from build123d import *

# Parameters (mm, degrees)
F3_D            = 5.5
F3_COPIES_COUNT = 6


# Not quite as in the source:
# - a pattern or mirror of a feature is missing from the dataset's text; its kind, count and spacing are read off the source's solid


with BuildPart() as f1:
    # F0 (on Front) → F1 (revolve)
    with BuildSketch(Plane.XZ):
        Polygon((-25, 16.5), (-25, 11), (25, 11), (25, 16.5), (4, 18), (4, 34), (-4, 34), (-4, 18), align=None)
    revolve(axis=Axis((-2.8921069455, 0, 0), (1, 0, 0)))

    # F3 (through all)
    with Locations(Plane.YZ.offset(4)):
        with Locations((0, 25)):
            f3 = Hole(F3_D / 2)

    # F3_copies: F3 ×6 about axis
    f3_copies_axis = Axis((0, 0, 0), (1, 0, 0))
    for i in range(1, F3_COPIES_COUNT):
        add(f3.rotate(f3_copies_axis, i * 360 / F3_COPIES_COUNT), mode=Mode.SUBTRACT)


solid = f1.part
Design review of the part built by this model. Coordinates are the model's own, in mm. A direction names the side the tool comes from. Give positions to 0.01 mm unless a question says otherwise; leave off trailing zeros. Loops run counter-clockwise (first coordinate to the right, second up) from the corner with the lowest first, then second, coordinate; pieces in that order, holes last. Notation, with made-up numbers: (33.5, -12.5) - (53.5, -12.5) arc R33 cw to (53.5, 24.5) - close; hole circle Ø2 at (8, 43.25). An arc over 180 degrees is marked (long way). Use CSV: the item, a comma, the result in double quotes. Start each with the question number.
1. Insertion check: P1, Ø9, axis at y = 0, z = -25, coming from the +X side; P2, Ø9, axis at y = 0, z = 25, coming from the -X side; P3, Ø3, axis at x = 11.5, z = 7, coming from the -Y side. Each pin has a flat end and moves straight along its axis. Give the tip position at first contact, or say it passes through.
2. Machinability: for faces 4 (the cylindrical face through (-0.056, 0.358, 27.727)), 5 (the flat face through (4, 15, -15)), which of the approach directions +Z, -Z, +X, -X, +Y, -Y give a long, thin tool a straight path to every point of the face, cutting with its end or side? Answer none if there is none.
3. Add section A-A (z = 0). State the section outline as (x, y) points.
4. Draft analysis for pull direction Z (two halves, no side actions). For faces 1 (the conical face through (16.686, -5.135, 16.304)), 2 (the cylindrical face through (-0.056, -0.358, -27.727)), 3 (the flat face through (-4, 15, 15)), state which applies: released by +Z, released by -Z, zero draft, split by the parting line, or undercut.
5. Add section C-C (x = 20). State the section outline as (y, z) points, plus the area to 3 significant figures.
6. Add section D-D (z = 25). State the section outline as (x, y) points, plus the area to 3 significant figures.
7. Wall thickness on L1, parallel to Y at x = 1, z = 12; L2, parallel to X at y = -5, z = -19.5; L3, parallel to Y at x = 22.5, z = -1.5: over which ranges is each line inside the solid? List them lowest first.
8. Add section B-B (y = 0). State the section outline as (x, z) points.
Results found:
1,P1,"stops at x = 4"
1,P2,"stops at x = -4"
1,P3,"stops at y = -16.59"
2,face 4,"+X, -X"
2,face 5,"+X"
3,outline,"(-25, -16.5) - (-4, -18) - (-4, -34) - (4, -34) - (4, -18) - (25, -16.5) - (25, -11) - (-25, -11) - close; (-25, 11) - (25, 11) - (25, 16.5) - (4, 18) - (4, 34) - (-4, 34) - (-4, 18) - (-25, 16.5) - close"
4,face 1,"split by the parting line"
4,face 2,"undercut"
4,face 3,"zero draft"
5,outline,"circle Ø33.71 at (0, 0); hole circle Ø22 at (0, 0)"
5,area,"513 mm²"
6,outline,"(-4, -23.04) - (4, -23.04) - (4, -2.75) - (-4, -2.75) - close; (-4, 2.75) - (4, 2.75) - (4, 23.04) - (-4, 23.04) - close"
6,area,"325 mm²"
7,L1,"y = -31.81 to -24.35, -18.95 to 18.95, 24.35 to 31.81"
7,L2,"x = -4 to 4"
7,L3,"y = -16.61 to -10.9, 10.9 to 16.61"
8,outline,"(-25, -16.5) - (-4, -18) - (-4, -22.25) - (4, -22.25) - (4, -18) - (25, -16.5) - (25, -11) - (-25, -11) - close; (-25, 11) - (25, 11) - (25, 16.5) - (4, 18) - (4, 22.25) - (-4, 22.25) - (-4, 18) - (-25, 16.5) - close; (-4, -34) - (4, -34) - (4, -27.75) - (-4, -27.75) - close; (-4, 27.75) - (4, 27.75) - (4, 34) - (-4, 34) - close"
